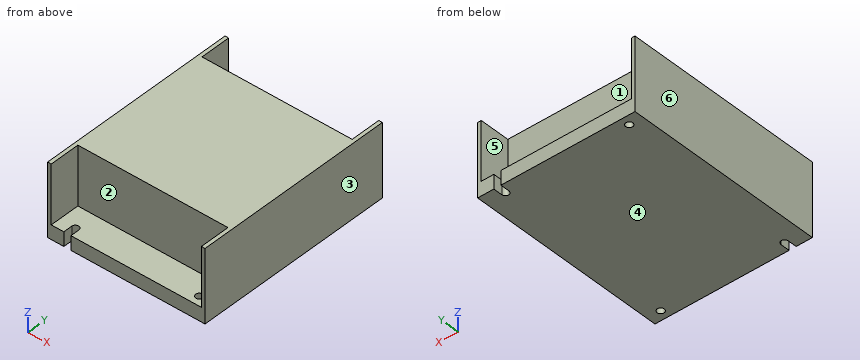
```python
from build123d import *

# Parameters (mm, degrees)
SKETCH_1_W          = 78
SKETCH_1_H          = 100
EXTRUDE_1_DEPTH     = 36
SKETCH_2_W          = 74.4
SKETCH_2_H          = 15
CUT_EXTRUDE_1_DEPTH = 29
SKETCH_4_R          = 1.75
CUT_EXTRUDE_2_DEPTH = 10


with BuildPart() as part:
    # 草图1 → 凸台-拉伸1 (new body)
    with BuildSketch(Plane.XY):
        Rectangle(SKETCH_1_W, SKETCH_1_H)
    extrude(amount=EXTRUDE_1_DEPTH)

    # 草图2 → 切除-拉伸1 (cut)
    with BuildSketch(Plane.XY.offset(36)):
        with Locations((0, 42.5)):
            Rectangle(SKETCH_2_W, SKETCH_2_H)
    cut_extrude_1 = extrude(amount=-CUT_EXTRUDE_1_DEPTH, mode=Mode.SUBTRACT)

    # 草图4 → 切除-拉伸2 (cut)
    with BuildSketch(Plane(origin=(0, 0, 0), x_dir=(-1, 0, 0), z_dir=(0, 0, -1))):
        with Locations((-32.199434729, -45.5)):
            Circle(SKETCH_4_R)
        with Locations((32.199434729, 45.5)):
            Circle(SKETCH_4_R)
        with BuildLine():
            Line((27.464507609, -45.5), (27.464507609, -50))
            Line((27.464507609, -50), (30.964507609, -50))
            Line((30.964507609, -50), (30.964507609, -45.5))
            ThreePointArc((30.964507609, -45.5), (29.214507609, -43.75), (27.464507609, -45.5))
        make_face()
        with BuildLine():
            Line((-27.464507609, 45.5), (-27.464507609, 50))
            Line((-27.464507609, 50), (-30.964507609, 50))
            Line((-30.964507609, 50), (-30.964507609, 45.5))
            ThreePointArc((-30.964507609, 45.5), (-29.214507609, 43.75), (-27.464507609, 45.5))
        make_face()
    extrude(amount=-CUT_EXTRUDE_2_DEPTH, mode=Mode.SUBTRACT)

    # 镜向1: 切除-拉伸1 across plane
    add(cut_extrude_1.mirror(Plane.ZX), mode=Mode.SUBTRACT)


solid = part.part
```
Geometry: final body of the model. Coordinates: model frame, mm. Face numbers are marked on the shaded views. A direction names the side the tool comes from. Give positions to 0.01 mm unless a question says otherwise; leave off trailing zeros. Loops run counter-clockwise (first coordinate to the right, second up) from the corner with the lowest first, then second, coordinate; pieces in that order, holes last. Notation, with made-up numbers: (82, 32.25) - (121, 32.25) arc R21 ccw to (121, 64.25) - close; hole circle Ø6 at (-19, -2.5). An arc over 180 degrees is marked (long way). Answer as CSV lines item,"result". Start each with the question number.
(1) Pin query (flat end, axial travel): P1, Ø1, axis at x = -4, y = -34.5, coming from the -Z side; P2, Ø4.5, axis at x = 16.5, y = 41, coming from the +Z side; P3, Ø8, axis at x = 4, z = 16, coming from the -Y side; P4, Ø1.5, axis at x = -1.5, z = 15, coming from the +Y side. Return the tip coordinate at first contact, or that it passes through.
(2) Section query B-B (x = -16.5). Output: boundary loops of the cut face in (y, z), and give its area (3 significant figures).
(3) Section query A-A (z = 33). Output: boundary loops of the cut face in (x, y), and give its area (3 significant figures).
(4) Ray query, line 1 along X through (y, z) = (-38, 30.5); line 2 along Z through (x, y) = (14, 42.5); line 3 along Y through (x, z) = (19, 23). Return the intervals inside material, ascending. Write a range as [from, to].
(5) Mould query, pull axis X, two halves, no side actions, for the marked faces 4, 5 and 6. Classes: +X half, -X half, draft (parallel to the pull), parting line (faces both ways), or undercut.
(6) Reachability of the marked faces 1, 2 and 3 from +Z, -Z, +X, -X, +Y, -Y: full face, straight path, thin tool, end or side. Return the list, or none.
Worked answers:
1,P1,"stops at z = 0"
1,P2,"stops at z = 7"
1,P3,"stops at y = -35"
1,P4,"stops at y = 35"
2,outline,"(-50, 0) - (50, 0) - (50, 7) - (35, 7) - (35, 36) - (-35, 36) - (-35, 7) - (-50, 7) - close"
2,area,"2,730 mm^2"
3,outline,"(-39, -50) - (-37.2, -50) - (-37.2, -35) - (37.2, -35) - (37.2, -50) - (39, -50) - (39, 50) - (37.2, 50) - (37.2, 35) - (-37.2, 35) - (-37.2, 50) - (-39, 50) - close"
3,area,"5,570 mm^2"
4,line 1,"x = [-39, -37.2], [37.2, 39]"
4,line 2,"z = [0, 7]"
4,line 3,"y = [-35, 35]"
5,face 4,"draft"
5,face 5,"undercut"
5,face 6,"-X half"
6,face 1,"+Z, +Y"
6,face 2,"+Z, -Y"
6,face 3,"+Z, -Z, +X, +Y, -Y"
